Design review of the part built by this model. Coordinates are the model's own, in mm. Face numbers are marked on the shaded views. A direction names the side the tool comes from. Coordinates: 2 decimals unless noted, no trailing zeros. Loops run counter-clockwise (first coordinate to the right, second up) from the corner with the lowest first, then second, coordinate; pieces in that order, holes last. Notation, with made-up numbers: (36, -32) - (75, -32) arc R31 ccw to (75, -7) - close; hole circle Ø4 at (77.25, 61). An arc over 180 degrees is marked (long way). Answer in a Markdown table with one row per item. Add a question column.
(1) The part is to be moulded in two halves that separate along X. For the marked faces 3, 4 and 5, say which applies: released by +X, released by -X, zero draft, split by the parting line, or undercut.
(2) We need section A-A, the plane y = -4. Write out the cut boundary in (x, z), plus the area to 3 significant figures.
(3) To check wall thickness, follow L1, parallel to X at y = 1, z = 2.5; L2, parallel to Y at x = -28.9, z = 5.6; L3, parallel to Y at x = 40, z = 6.75. State the ranges of each line that lie inside material, in increasing order. Write a range as [from, to].
(4) Clearance check with flat-ended pins moving along their axes: pin 1 (1 mm diameter, centred on x = 62.5, y = -28.5, fed in from +Z); pin 2 (2.5 mm diameter, centred on x = -28, z = 3, fed in from -Y); pin 3 (1 mm diameter, centred on y = 27, z = 6.5, fed in from -X). State where each tip first meets the part, or that it passes through.
(5) We need section B-B, the plane z = 1.75. Give the number of separate pieces and of enclosed holes in the cut face, plus the area to 3 significant figures.
(6) For the marked faces 1 and 2, list the 3-axis set-ups (+Z, -Z, +X, -X, +Y, -Y) from which the entire face can be reached by the end or side of a thin tool; tool diameter is ignored.
(7) We need section C-C, the plane y = 48. Write out the cut boundary in (x, z).
from build123d import *

# Parameters (mm, degrees)
F0_R     = 1
F0_W     = 12.8
F0_H     = 4.05
F1_DEPTH = 9
F2_DEPTH = 4


with BuildPart() as f1:
    # F0 (on Top) → F1 (new body)
    with BuildSketch(Plane.XY):
        Polygon((-40, -21), (-40, -25), (-32.387223, -33.881573), (-28.818717, -30.822853), (-19.100233, -22.492724), (-16.464528, -25.567713), (-0.650297, -44.017649), (1.985408, -47.092638), (-7.733077, -55.422767), (-11.301583, -58.481487), (-10, -60), (20, -60), (20, 60), (-10, 60), (-16.311194, 52.63694), (-12.742688, 49.578221), (-3.024203, 41.248091), (-5.659909, 38.173102), (-21.474139, 19.723167), (-24.109844, 16.648177), (-33.828328, 24.978307), (-37.396835, 28.037026), (-40, 25), (-40, 11.4), (-35.3, 11.4), (-22.5, 11.4), (-22.5, 7.35), (-22.5, -16.95), (-22.5, -21), (-35.3, -21), align=None)
        with Locations((0, -29)):
            Circle(F0_R, mode=Mode.SUBTRACT)
        with Locations((0, 30)):
            Circle(F0_R, mode=Mode.SUBTRACT)
        with Locations((10, 55)):
            Circle(F0_R, mode=Mode.SUBTRACT)
        Polygon((-40, 11.4), (-40, -21), (-35.3, -21), (-35.3, -16.95), (-35.3, 7.35), (-35.3, 11.4), align=None)
        Polygon((-28.818717, -30.822853), (-32.387223, -33.881573), (-11.301583, -58.481487), (-7.733077, -55.422767), (-10.368782, -52.347778), (-26.183012, -33.897843), align=None)
        Polygon((-16.311194, 52.63694), (-37.396835, 28.037026), (-33.828328, 24.978307), (-31.192623, 28.053296), (-15.378393, 46.503232), (-12.742688, 49.578221), align=None)
        Polygon((-10.368782, -52.347778), (-7.733077, -55.422767), (1.985408, -47.092638), (-0.650297, -44.017649), align=None)
        with Locations((-4.500813, -49.359561)):
            Circle(F0_R, mode=Mode.SUBTRACT)
        Polygon((-19.100233, -22.492724), (-28.818717, -30.822853), (-26.183012, -33.897843), (-16.464528, -25.567713), align=None)
        with Locations((-22.332497, -28.55593)):
            Circle(F0_R, mode=Mode.SUBTRACT)
        with Locations((-28.9, -18.975)):
            Rectangle(F0_W, F0_H)
        with Locations((-28.9, -18.5)):
            Circle(F0_R, mode=Mode.SUBTRACT)
        with Locations((-28.9, 9.375)):
            Rectangle(F0_W, F0_H)
        with Locations((-28.9, 8.9)):
            Circle(F0_R, mode=Mode.SUBTRACT)
        Polygon((-3.024203, 41.248091), (-12.742688, 49.578221), (-15.378393, 46.503232), (-5.659909, 38.173102), align=None)
        with Locations((-9.510424, 43.515015)):
            Circle(F0_R, mode=Mode.SUBTRACT)
        Polygon((-31.192623, 28.053296), (-33.828328, 24.978307), (-24.109844, 16.648177), (-21.474139, 19.723167), align=None)
        with Locations((-27.342108, 22.711384)):
            Circle(F0_R, mode=Mode.SUBTRACT)
    extrude(amount=F1_DEPTH)

    # F0 (on Top) → F2 (join)
    with BuildSketch(Plane.XY):
        with Locations((-9.510424, 43.515015)):
            Circle(F0_R)
        with Locations((-27.342108, 22.711384)):
            Circle(F0_R)
        with Locations((-28.9, 8.9)):
            Circle(F0_R)
        with Locations((-28.9, -18.5)):
            Circle(F0_R)
        with Locations((-22.332497, -28.55593)):
            Circle(F0_R)
        with Locations((-4.500813, -49.359561)):
            Circle(F0_R)
    extrude(amount=F2_DEPTH)

    # F3: F1 across face


with BuildPart() as f1_1:
    add(f1.part)
    add(f1.part.mirror(Plane(origin=(20, 0, 4.5), x_dir=(0, 1, 0), z_dir=(1, 0, 0))))


solid = f1_1.part
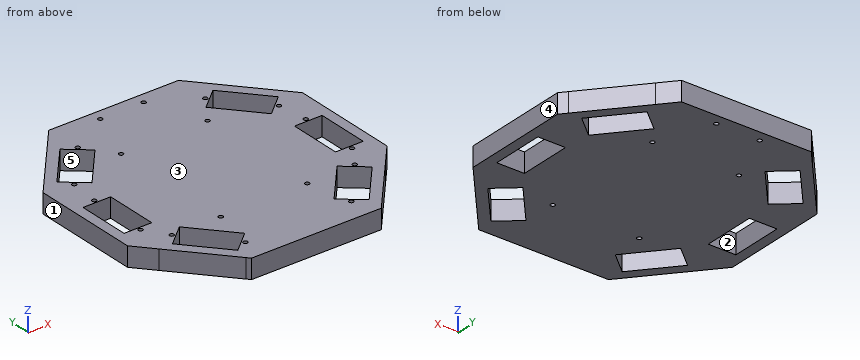
Responses:
| question | item | result |
|---|---|---|
| 1 | face 3 | zero draft |
| 1 | face 4 | released by +X |
| 1 | face 5 | undercut |
| 2 | outline | (-40, 0) - (-35.3, 0) - (-35.3, 9) - (-40, 9) - close; (-22.5, 0) - (62.5, 0) - (62.5, 9) - (-22.5, 9) - close; (75.3, 0) - (80, 0) - (80, 9) - (75.3, 9) - close |
| 2 | area | 850 mm2 |
| 3 | L1 | x = [-40, -35.3], [-22.5, 62.5], [75.3, 80] |
| 3 | L2 | y = [-37.95, -19.5], [-17.5, -16.95], [7.35, 7.9], [9.9, 26.09], [30.73, 37.95] |
| 3 | L3 | y = [-60, -30], [-28, 29], [31, 60] |
| 4 | pin 1 | stops at z = 4 |
| 4 | pin 2 | stops at y = -40.46 |
| 4 | pin 3 | stops at x = -38.71 |
| 5 | separate pieces | 1 |
| 5 | enclosed holes | 12 |
| 5 | area | 10,400 mm2 |
| 6 | face 1 | +Z, -Z, -X, +Y, -Y |
| 6 | face 2 | +Z, -Z |
| 7 | outline | (-20.29, 0) - (60.29, 0) - (60.29, 9) - (-20.29, 9) - close |
